Verification items for this drawing (mm, ordinates from the low corner). Give positions to 0.01 mm unless a question says otherwise; leave off trailing zeros. Loops run counter-clockwise (first coordinate to the right, second up) from the corner with the lowest first, then second, coordinate; pieces in that order, holes last. Notation, with made-up numbers: (77.25, 3) -> (99.25, 3) arc R19 cw to (99.25, 14) -> close; hole circle Ø3 at (84, -27.75). An arc over 180 degrees is marked (long way). Answer in a Markdown table with one row per item. Add a question column.
Q1. Material ranges on probe 1 along X at (y, z) = (29, 0.55); probe 2 along Y at (x, z) = (13.5, 1.2); probe 3 along Y at (x, z) = (17, 0.55), recorded low to high.
Q2. Section check A-A on y = 125.5. Enter the section's corners in (x, z).
Q3. Gauge pin test, flat ends, axial feed: P1, Ø2.5, axis at y = 27, z = 2.5, coming from the -X side; P2, Ø9.5, axis at x = 230.39, y = 75, coming from the +Z side; P3, Ø3, axis at y = 88.5, z = 3, coming from the +X side; P4, Ø3, axis at x = 33, y = 113, coming from the -Z side. Record the tip position at first contact, or that the pin passes through.
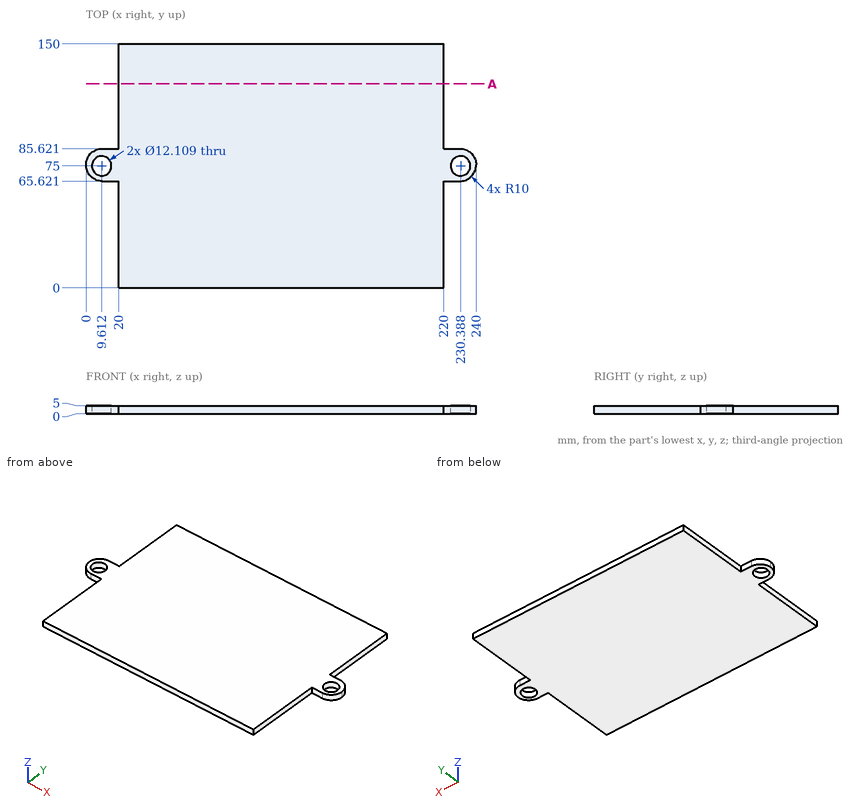
Taken from the geometry:
| question | item | result |
|---|---|---|
| 1 | probe 1 | x = 20 to 220 |
| 1 | probe 2 | y = 65.62 to 70.36, 79.64 to 85.62 |
| 1 | probe 3 | y = 65.62 to 85.62 |
| 2 | outline | (20, 0) -> (220, 0) -> (220, 5) -> (20, 5) -> close |
| 3 | P1 | stops at x = 20 |
| 3 | P2 | passes through |
| 3 | P3 | stops at x = 220 |
| 3 | P4 | stops at z = 0 |
